```python
from build123d import *

# Parameters (mm, degrees)
SALIENTE_EXTRUIR1_DEPTH = 40
CROQUIS2_R              = 11
SALIENTE_EXTRUIR2_DEPTH = 2
CROQUIS3_R              = 5
CORTAR_EXTRUIR1_DEPTH   = 3.5
CROQUIS4_R              = 2.5
SALIENTE_EXTRUIR3_DEPTH = 25.5
CROQUIS5_R              = 2
CORTAR_EXTRUIR2_DEPTH   = 4.5
CORTAR_EXTRUIR3_START   = -17.5
CORTAR_EXTRUIR3_DEPTH   = 17.5
CORTAR_EXTRUIR4_START   = -8
CORTAR_EXTRUIR4_DEPTH   = 22.5
CROQUIS8_W              = 16.5
CROQUIS8_H              = 9.5
SALIENTE_EXTRUIR4_DEPTH = 5


with BuildPart() as part:
    # Croquis1 → Saliente-Extruir1 (new body)
    with BuildSketch(Plane.XY):
        Polygon((-17.614466094, -21.15), (17.614466094, -21.15), (21.15, -17.614466094), (21.15, 17.614466094), (17.614466094, 21.15), (-17.614466094, 21.15), (-21.15, 17.614466094), (-21.15, -17.614466094), align=None)
    extrude(amount=-SALIENTE_EXTRUIR1_DEPTH)

    # Croquis2 → Saliente-Extruir2 (add)
    with BuildSketch(Plane.XY):
        Circle(CROQUIS2_R)
    extrude(amount=SALIENTE_EXTRUIR2_DEPTH)

    # Croquis3 → Cortar-Extruir1 (cut)
    with BuildSketch(Plane.XY.offset(2)):
        Circle(CROQUIS3_R)
    extrude(amount=-CORTAR_EXTRUIR1_DEPTH, mode=Mode.SUBTRACT)

    # Croquis4 → Saliente-Extruir3 (add)
    with BuildSketch(Plane.XY.offset(-1.5)):
        Circle(CROQUIS4_R)
    extrude(amount=SALIENTE_EXTRUIR3_DEPTH)

    # Croquis5 → Cortar-Extruir2 (cut)
    with BuildSketch(Plane.XY):
        with Locations((-15.5, 15.5)):
            Circle(CROQUIS5_R)
        with Locations((15.5, 15.5)):
            Circle(CROQUIS5_R)
        with Locations((15.5, -15.5)):
            Circle(CROQUIS5_R)
        with Locations((-15.5, -15.5)):
            Circle(CROQUIS5_R)
    extrude(amount=-CORTAR_EXTRUIR2_DEPTH, mode=Mode.SUBTRACT)

    # Croquis6 → Cortar-Extruir3 (cut)
    with BuildSketch(Plane.XY.offset(24).offset(CORTAR_EXTRUIR3_START)):
        with BuildLine():
            Line((-1.5, 2), (1.5, 2))
            ThreePointArc((1.5, 2), (0, 2.5), (-1.5, 2))
        make_face()
    extrude(amount=CORTAR_EXTRUIR3_DEPTH, mode=Mode.SUBTRACT)

    # Croquis7 → Cortar-Extruir4 (cut)
    with BuildSketch(Plane.XY.offset(CORTAR_EXTRUIR4_START)):
        Polygon((-21.15, 12.15), (-12.15, 21.15), (-21.15, 21.15), align=None)
        Polygon((21.15, 21.15), (21.15, 12.15), (12.15, 21.15), align=None)
        Polygon((21.15, -21.15), (21.15, -12.15), (12.15, -21.15), align=None)
        Polygon((-21.15, -12.15), (-12.15, -21.15), (-21.15, -21.15), align=None)
    extrude(amount=-CORTAR_EXTRUIR4_DEPTH, mode=Mode.SUBTRACT)

    # Croquis8 → Saliente-Extruir4 (add)
    with BuildSketch(Plane(origin=(0, 21.15, 0), x_dir=(1, 0, 0), z_dir=(0, 1, 0))):
        with Locations((0, 35.25)):
            Rectangle(CROQUIS8_W, CROQUIS8_H)
    extrude(amount=SALIENTE_EXTRUIR4_DEPTH)


solid = part.part
```
Verification items for the finished model (mm, model axes). A direction names the side the tool comes from. Round coordinates to 2 decimals unless told otherwise and drop trailing zeros. Write each loop counter-clockwise with the first axis right and the second up, starting at its lowest first coordinate (ties: lowest second). Pieces come first, ordered by that corner, then holes. Notation, with made-up numbers: (73, 9) -> (77, 9) arc R29 cw to (77, 48) -> close; hole circle Ø8 at (0.5, 19.5). An arc over 180 degrees is marked (long way). Write each question's results on one line, items separated by ' | '.
Q1. Go/stop test with flat-tipped pins: pin 1 Ø7 at (x, y) = (17, 18.5) entering from +Z; pin 2 Ø10.5 at (x, z) = (-3.5, -23) entering from +Y; pin 3 Ø1.2 at (x, y) = (15.5, -16.5) entering from +Z. Record where each tip stops, or that it passes through.
Derived:
pin 1: stops at z = 0 | pin 2: stops at y = 21.15 | pin 3: stops at z = -4.5
Q2. Thickness scan on probe 1 along Y at (x, z) = (-15.5, -1.95); probe 2 along Y at (x, z) = (15, -1); probe 3 along Z at (x, y) = (-17.5, 17.5). Record the ranges inside material, lowest first.
Derived:
probe 1: y = -21.15 to -17.5, -13.5 to 13.5, 17.5 to 21.15 | probe 2: y = -21.15 to -17.44, -13.56 to 13.56, 17.44 to 21.15 | probe 3: z = -40 to -30.5, -8 to 0
Q3. Sectioned sample at B-B, the plane y = 0. Record the boundary of the cut face in (x, z), and give its area (3 significant figures).
Derived:
outline: (-21.15, -40) -> (21.15, -40) -> (21.15, 0) -> (11, 0) -> (11, 2) -> (5, 2) -> (5, -1.5) -> (2.5, -1.5) -> (2.5, 24) -> (-2.5, 24) -> (-2.5, -1.5) -> (-5, -1.5) -> (-5, 2) -> (-11, 2) -> (-11, 0) -> (-21.15, 0) -> close | area: 1,830 mm²
Q4. Sectioned sample at D-D, the plane x = 0. Record the boundary of the cut face in (y, z).
Derived:
outline: (-21.15, -40) -> (26.15, -40) -> (26.15, -30.5) -> (21.15, -30.5) -> (21.15, 0) -> (11, 0) -> (11, 2) -> (5, 2) -> (5, -1.5) -> (2.5, -1.5) -> (2.5, 6.5) -> (2, 6.5) -> (2, 24) -> (-2.5, 24) -> (-2.5, -1.5) -> (-5, -1.5) -> (-5, 2) -> (-11, 2) -> (-11, 0) -> (-21.15, 0) -> close
Q5. Access from +Z, -Z, +X, -X, +Y, -Y to the whole of each face (thin tool, end or side, straight path). Record for faces 4 (the face through (18, 18, -30.5)), 5 (the face through (0, 2, 15)), 6 (the face through (-8.25, 24, -35)), 7 (the face through (15, 16, -4.5)), 8 (the face through (-18, 18, -8)).
Derived:
face 4: +X, +Y | face 5: +Z, +X, -X, +Y | face 6: +Z, -Z, -X, +Y | face 7: +Z | face 8: -X, +Y
Q6. Sectioned sample at C-C, the plane z = -5.5. Record the boundary of the cut face in (x, y), and give its area (3 significant figures).
Derived:
outline: (-21.15, -17.61) -> (-17.61, -21.15) -> (17.61, -21.15) -> (21.15, -17.61) -> (21.15, 17.61) -> (17.61, 21.15) -> (-17.61, 21.15) -> (-21.15, 17.61) -> close | area: 1,760 mm²
Q7. Draft check along Y on faces 1 (the face through (21.15, 0, -20)), 2 (the face through (-16, 16, -4.5)), 3 (the face through (-16.7, -16.6, -19.1)). Enter one of: released by +Y, released by -Y, zero draft, split by the parting line, or undercut.
Derived:
face 1: zero draft | face 2: undercut | face 3: released by -Y
Q8. Sectioned sample at A-A, the plane x = -15.5. Record the boundary of the cut face in (y, z), and give its area (3 significant figures).
Derived:
outline: (-21.15, -40) -> (21.15, -40) -> (21.15, -30.5) -> (17.8, -30.5) -> (17.8, -8) -> (21.15, -8) -> (21.15, 0) -> (17.5, 0) -> (17.5, -4.5) -> (13.5, -4.5) -> (13.5, 0) -> (-13.5, 0) -> (-13.5, -4.5) -> (-17.5, -4.5) -> (-17.5, 0) -> (-21.15, 0) -> (-21.15, -8) -> (-17.8, -8) -> (-17.8, -30.5) -> (-21.15, -30.5) -> close | area: 1,510 mm²
